Source: CAD feature listing. Evaluate the final solid. Frame: model axes, mm. Face numbers are marked on the shaded views. Give positions to 0.01 mm unless a question says otherwise; leave off trailing zeros. Loops run counter-clockwise (first coordinate to the right, second up) from the corner with the lowest first, then second, coordinate; pieces in that order, holes last. Notation, with made-up numbers: M 11,51 L 51,51 A18 cw 51,80 Z; hole C 66,48.5 d7. An arc over 180 degrees is marked long. Answer in a Markdown table with one row per item.
```python
from build123d import *

# Parameters (mm, degrees)
BOSS_EXTRUDE2_DEPTH        = 3.175
F_10_32_TAPPED_HOLE2_D     = 4.0386
F_10_32_TAPPED_HOLE2_DEPTH = 6.35
CHAMFER4_SIZE              = 0.762
CHAMFER5_SIZE              = 0.508


with BuildPart() as part:
    # Sketch10 → Boss-Extrude2 (new body, symmetric)
    with BuildSketch(Plane(origin=(0, 0, 0), x_dir=(1, 0, 0), z_dir=(0, 1, 0))):
        with BuildLine():
            Line((-19.05, 9.525), (19.05, 9.525))
            ThreePointArc((19.05, 9.525), (28.575, 0), (19.05, -9.525))
            Line((19.05, -9.525), (-19.05, -9.525))
            ThreePointArc((-19.05, -9.525), (-28.575, 0), (-19.05, 9.525))
        make_face()
    extrude(amount=BOSS_EXTRUDE2_DEPTH, both=True)

    # #10-32 Tapped Hole2
    with Locations(Plane(origin=(0, 3.175, 0), x_dir=(1, 0, 0), z_dir=(0, 1, 0))):
        with Locations((19.05, 0), (-19.05, 0), (0, 0)):
            Hole(F_10_32_TAPPED_HOLE2_D / 2, depth=F_10_32_TAPPED_HOLE2_DEPTH)

    # Chamfer4
    chamfer4_edges = [part.edges().sort_by_distance(p)[0] for p in [
        (28.575, 3.175, 0),
        (0, 3.175, -9.525),
        (-28.575, 3.175, 0),
        (0, -3.175, -9.525),
        (28.575, -3.175, 0),
        (0, -3.175, 9.525),
        (-28.575, -3.175, 0),
        (0, 3.175, 9.525),
    ]]
    chamfer(chamfer4_edges, length=CHAMFER4_SIZE)

    # Chamfer5
    chamfer5_edges = [part.edges().sort_by_distance(p)[0] for p in [
        (2.0193, 3.175, 0),
        (2.0193, -3.175, 0),
        (-17.0307, 3.175, 0),
        (-17.0307, -3.175, 0),
        (21.0693, 3.175, 0),
        (21.0693, -3.175, 0),
    ]]
    chamfer(chamfer5_edges, length=CHAMFER5_SIZE)


solid = part.part
```
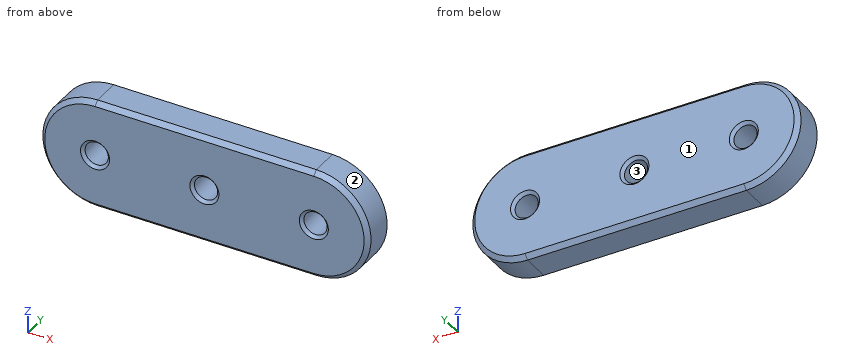
1) Material intervals for L1, parallel to X at y = 0.45, z = 0 (3 decimals); L2, parallel to Z at x = 0, y = -1.4 (3 decimals); L3, parallel to X at y = 0.25, z = -1, sorted ascending.
Reply:
| item | result |
|---|---|
| L1 | x = -28.575 to -21.069, -17.031 to -2.019, 2.019 to 17.031, 21.069 to 28.575 |
| L2 | z = -9.525 to -2.019, 2.019 to 9.525 |
| L3 | x = -28.52 to -20.8, -17.3 to -1.75, 1.75 to 17.3, 20.8 to 28.52 |
2) Section C-C, the plane y = 1.5. Return loops of the section in (x, z) (3 decimals).
Reply:
| item | result |
|---|---|
| outline | M -19.05,-9.525 L 19.05,-9.525 A9.525 ccw 19.05,9.525 L -19.05,9.525 A9.525 ccw Z; hole C -19.05,0 d4.039; hole C 0,0 d4.039; hole C 19.05,0 d4.039 |
3) Pin query (flat end, axial travel): pin 1 Ø3 at (y, z) = (-1, 4) entering from -X; pin 2 Ø1.5 at (y, z) = (0.5, 2) entering from -X; pin 3 Ø4.5 at (x, z) = (-19.05, 0) entering from -Y. Return the tip coordinate at first contact, or that it passes through.
Reply:
| item | result |
|---|---|
| pin 1 | stops at x = -28.24 |
| pin 2 | stops at x = -28.49 |
| pin 3 | stops at y = -2.9 |
4) Pull-direction query (Z, two-part tool) for the marked faces 1, 2 and 3; classes: released by +Z, released by -Z, zero draft, split by the parting line, or undercut.
Reply:
| item | result |
|---|---|
| face 1 | zero draft |
| face 2 | split by the parting line |
| face 3 | undercut |
5) Section A-A, the plane z = 0. Count the separate pieces of the cut face and the enclosed holes in it, then the cut area to 3 significant figures.
Reply:
| item | result |
|---|---|
| separate pieces | 4 |
| enclosed holes | 0 |
| area | 283 mm² |
6) Section B-B, the plane x = 0. Return loops of the section in (y, z) (3 decimals).
Reply:
| item | result |
|---|---|
| outline | M -3.175,-8.763 L -2.413,-9.525 L 2.413,-9.525 L 3.175,-8.763 L 3.175,-2.527 L 2.667,-2.019 L -2.667,-2.019 L -3.175,-2.527 Z; M -3.175,2.527 L -2.667,2.019 L 2.667,2.019 L 3.175,2.527 L 3.175,8.763 L 2.413,9.525 L -2.413,9.525 L -3.175,8.763 Z |
